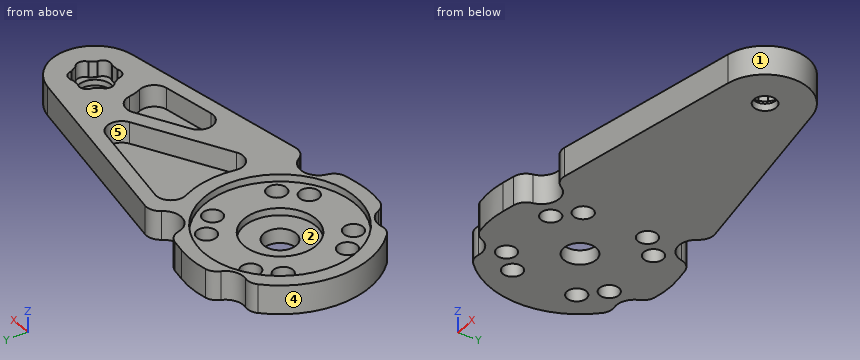
Autodesk Inventor part; units mm, degrees
ref_plane "YZ Plane" through (0, 0, 0) normal (1, 0, 0) x (0, 1, 0)
ref_plane "XZ Plane" through (0, 0, 0) normal (0, 1, 0) x (-1, 0, 0)
ref_plane "XY Plane" through (0, 0, 0) normal (0, 0, 1) x (1, 0, 0)
sketch "スケッチ1" plane through (0, 0, 0) normal (0, 0, 1) x (1, 0, 0)
  circle A0 centre (0, 0) radius 10.5 construction
  circle A1 centre (0, 0) radius 5 construction
  circle A2 centre (0, 0) radius 5.01
  circle A3 centre (0, 0) radius 10.51
  arc A4 (2.1531, 12.3132) -> (2.1531, -12.3132) centre (0, 0) ccw
  circle A5 centre (37.7359, 0) radius 2.25
  arc A6 (38.7694, -5.9103) -> (38.7694, 5.9103) centre (37.7359, 0) ccw
  line L0 (2.1531, 12.3132) -> (38.7694, 5.9103)
  line L1 (2.1531, -12.3132) -> (38.7694, -5.9103)
  line L2 (13.3804, 8.3196) -> (26.7879, 5.9751)
  line L3 (30.7947, -5.2745) -> (23.5904, -6.5342)
  arc A7 (2.1531, -12.3132) -> (-4.7001, 11.5827) centre (0, 0) ccw construction
  arc A8 (38.7694, 5.9103) -> (32.2717, -2.4783) centre (37.7359, 0) ccw construction
  line L4 (34.0196, 4.7105) -> (8.4896, -9.1748) construction
  line L5 (27.399, 2.248) -> (15.2168, -4.3777)
  line L6 (28.8431, 0.7568) -> (22.2903, -2.8072)
  line L7 (32.4358, 4.9875) -> (34.0196, 4.7105) construction
  line L8 (11.5743, -8.6354) -> (8.4896, -9.1748) construction
  arc A9 (31.783, -0.7501) -> (32.2717, -2.4783) centre (37.7359, 0) ccw
  arc A10 (12.2941, -2.2592) -> (11.2378, 5.4737) centre (0, 0) ccw
  line L9 (40.9229, 0) -> (40.3979, -0.9093) construction
  line L10 (39.3294, -2.76) -> (38.2794, -2.76) construction
  line L11 (36.1424, -2.76) -> (35.6174, -1.8507) construction
  line L12 (34.549, 0) -> (35.074, 0.9093) construction
  line L13 (36.1424, 2.76) -> (37.1924, 2.76) construction
  line L14 (39.3294, 2.76) -> (39.8544, 1.8507)
  arc A11 (40.3979, -0.9093) -> (40.3979, 0.9093) centre (39.8729, 0) ccw
  arc A12 (39.8544, 1.8507) -> (38.2794, 2.76) centre (38.8044, 1.8507) ccw
  arc A13 (37.1924, 2.76) -> (35.6174, 1.8507) centre (36.6674, 1.8507) ccw
  arc A14 (35.074, 0.9093) -> (35.074, -0.9093) centre (35.599, 0) ccw
  arc A15 (35.6174, -1.8507) -> (37.1924, -2.76) centre (36.6674, -1.8507) ccw
  arc A16 (38.2794, -2.76) -> (39.8544, -1.8507) centre (38.8044, -1.8507) ccw
  line L15 (40.3979, -0.9093) -> (39.8544, -1.8507)
  line L16 (39.8544, -1.8507) -> (39.3294, -2.76) construction
  line L17 (38.2794, -2.76) -> (37.1924, -2.76)
  line L18 (37.1924, -2.76) -> (36.1424, -2.76) construction
  line L19 (35.6174, -1.8507) -> (35.074, -0.9093)
  line L20 (35.074, -0.9093) -> (34.549, 0) construction
  line L21 (35.6174, 1.8507) -> (36.1424, 2.76) construction
  line L22 (35.074, 0.9093) -> (35.6174, 1.8507)
  line L23 (37.1924, 2.76) -> (38.2794, 2.76)
  line L24 (38.2794, 2.76) -> (39.3294, 2.76) construction
  line L25 (39.8544, 1.8507) -> (40.3979, 0.9093)
  line L26 (40.3979, 0.9093) -> (40.9229, 0) construction
  circle A17 centre (37.7359, 0) radius 1.55
  circle A18 centre (0, 0) radius 2.25
  line L27 (0, 0) -> (27.1359, -16.96) construction
  line L28 (37.7359, 0) -> (27.1359, -16.96) construction
  line L29 (0, 0) -> (37.7359, 0) construction
  line L30 (0, 0) -> (0.848, -0.53)
  line L31 (8.003, 10.918) -> (-6.307, -11.978) construction
  arc A19 (-3.808, -11.9058) -> (-7.6616, -9.8768) centre (-6.307, -11.978) ccw
  arc A20 (5.6301, 11.7052) -> (10.5021, 10.8532) centre (8.003, 10.918) ccw
  arc A21 (13.3804, 8.3196) -> (11.2378, 5.4737) centre (13.0359, 6.3495) ccw
  arc A22 (12.2941, -2.2592) -> (15.2168, -4.3777) centre (14.2612, -2.6207) ccw
  arc A23 (22.2903, -2.8072) -> (23.5904, -6.5342) centre (23.2459, -4.5641) ccw
  arc A24 (30.7947, -5.2745) -> (32.2717, -2.4783) centre (30.4502, -3.3043) ccw
  arc A25 (31.783, -0.7501) -> (28.8431, 0.7568) centre (29.7987, -1.0002) ccw
  arc A26 (27.399, 2.248) -> (26.7879, 5.9751) centre (26.4434, 4.005) ccw
  line L32 (8.003, -10.918) -> (-6.307, 11.978) construction
  arc A27 (-7.6616, 9.8768) -> (-3.808, 11.9058) centre (-6.307, 11.978) ccw
  arc A28 (10.5021, -10.8532) -> (5.6301, -11.7052) centre (8.003, -10.918) ccw
  line L33 (-6.625, -10.6) -> (6.625, 10.6) construction
  circle A29 centre (4.505, 7.208) radius 1.35
  circle A30 centre (-7.208, 4.505) radius 1.35
  circle A31 centre (-4.505, -7.208) radius 1.35
  circle A32 centre (7.208, -4.505) radius 1.35
  circle A33 centre (4.505, -7.208) radius 1.35
  circle A34 centre (-7.208, -4.505) radius 1.35
  circle A35 centre (-4.505, 7.208) radius 1.35
  circle A36 centre (7.208, 4.505) radius 1.35
  point P0 (8.4896, 9.1748)
  point P1 (34.0196, -4.7105)
  point P2 (10.3333, -7.0337)
  point P3 (32.3635, 2.6714)
  point P4 (39.3294, 2.76)
  point P5 (9.5861, 8.9831)
  point P6 (9.0332, 8.6401)
  point P7 (-3.808, 11.9058)
  dimension "d0" = 21
  dimension "d1" = 10
  dimension "d2" = 0.01
  dimension "d3" = 0.01
  dimension "d4" = 25
  dimension "d7" = 4.5
  dimension "d8" = 6
  dimension "d15" = 2
  dimension "d16" = 2
  dimension "d17" = 1
  dimension "d18" = 1
  dimension "d20" = 1.05
  dimension "d23" = 360
  dimension "d25" = 5.52
  dimension "d30" = 3.1
  dimension "d33" = 4.5
  dimension "d41" = 20
  dimension "d42" = 32
  dimension "d46" = 27
  dimension "d47" = 1
  dimension "d48" = 90
  dimension "d49" = 2.5
  dimension "d50" = 2.5
  dimension "d51" = 2
  dimension "d52" = 2
  dimension "d53" = 2
  dimension "d55" = 2.5
  dimension "d56" = 2.5
  dimension "d57" = 2.7
  dimension "d58" = 8.5
  dimension "d61" = 360
extrude "押し出し1" add sketch "スケッチ1" along normal blind 4 contours L0 A20 A6 L1 A28 A4 A19 A27
extrude "押し出し2" add sketch "スケッチ1" along normal blind 1.8 contours A12 L14 | L14 L25 A11 L15 A16 L17 A15 L19 A14 L22 A13 L23 A12
extrude "押し出し3" add sketch "スケッチ1" along normal blind 1 contours A5
extrude "押し出し4" add sketch "スケッチ1" along normal blind 3 contours A3
extrude "押し出し5" add sketch "スケッチ1" along normal blind 2 contours A2
extrude "押し出し6" add sketch "スケッチ1" along normal blind 1 contours L2 A26 L5 A22 A10 A21 | L3 A23 L6 A25 A9 A24
fillet "フィレット2" radius 2 8 edges at (-3.808, -11.9058, 2) (-7.6616, -9.8768, 2) (10.5021, 10.8532, 2) (5.6301, 11.7052, 2) (5.6301, -11.7052, 2) (10.5021, -10.8532, 2) (-7.6616, 9.8768, 2) (-3.808, 11.9058, 2)
equation "\"d3\" = d2"
equation "\"d18\" = d17"
equation "\"d50\" = d49"
properties part number "Ankle_side_pitch_frame" material "アルミニウム 2014-T4"
Read the model definition and answer for the solid it produces. Units are mm, in the model's axes. Face numbers are marked on the shaded views. A direction names the side the tool comes from. Coordinates: 2 decimals unless noted, no trailing zeros. Loops run counter-clockwise (first coordinate to the right, second up) from the corner with the lowest first, then second, coordinate; pieces in that order, holes last. Notation, with made-up numbers: (-24.75, 36) -> (14.25, 36) arc R21 cw to (14.25, 48) -> close; hole circle Ø8 at (-16.5, 24). An arc over 180 degrees is marked (long way). Write item = value, one per line. Start each with the question number.
1) The mould has two halves that part along X. Classify the marked faces 1, 2 and 3: pulls with the +X half, pulls with the -X half, needs draft (parallel to the pull), parting line crosses it, or undercut.
2) The part is cut by section A-A, the plane x = 0. Determine the outline of the cut face in (y, z).
3) For the marked faces 4 and 5, determine the directions among +Z, -Z, +X, -X, +Y, -Y from which every point of the face is accessible in a straight line to the end or side of a thin tool.
4) Find the intervals of material crossed by L1, parallel to X at y = 1.75, z = 1.5 (3 decimals); L2, parallel to Y at x = 27, z = 3.5; L3, parallel to Y at x = 0, z = 1.35, in increasing order. Write a range as from..to.
5) The part is cut by section B-B, the plane y = 0. State how many separate pieces and enclosed holes the cut face has, plus the area to 3 significant figures.
6) Given P1, Ø5, axis at x = 38, y = 0, coming from the +Z side; P2, Ø4, axis at x = 22.5, y = 2.5, coming from the +Z side; P3, Ø2, axis at y = -7.5, z = 2, coming from the -X side, each flat-ended and moving along its own axis, determine where each tip first touches the part or whether it passes through.
Result:
q1.face_1 = pulls with the +X half
q1.face_2 = undercut
q1.face_3 = needs draft
q2.outline = (-12.5, 0) -> (-2.25, 0) -> (-2.25, 2) -> (-5.01, 2) -> (-5.01, 3) -> (-10.51, 3) -> (-10.51, 4) -> (-12.5, 4) -> close; (2.25, 0) -> (12.5, 0) -> (12.5, 4) -> (10.51, 4) -> (10.51, 3) -> (5.01, 3) -> (5.01, 2) -> (2.25, 2) -> close
q3.face_4 = +Z, -Z, -X
q3.face_5 = +Z
q4.L1 = -12.377..-1.414, 1.414..12.377, 26.483..36.322, 39.15..43.475
q4.L2 = -7.97..-5.94, -0.25..2.03, 5.93..7.97
q4.L3 = -12.5..-2.25, 2.25..12.5
q5.separate_pieces = 3
q5.enclosed_holes = 0
q5.area = 120 mm²
q6.P1 = 1.8
q6.P2 = 1
q6.P3 = -10.68
